Could you check a few things on this model? Use its own coordinates, in mm. Face numbers are marked on the shaded views. A direction names the side the tool comes from. Give positions to 0.01 mm unless a question says otherwise; leave off trailing zeros. Write each loop counter-clockwise with the first axis right and the second up, starting at its lowest first coordinate (ties: lowest second). Pieces come first, ordered by that corner, then holes. Notation, with made-up numbers: (33.5, 25) - (77.5, 25) arc R27 cw to (77.5, 42) - close; hole circle Ø7 at (29.25, 32.5). An arc over 180 degrees is marked (long way). Use one line per item in the form item = value.
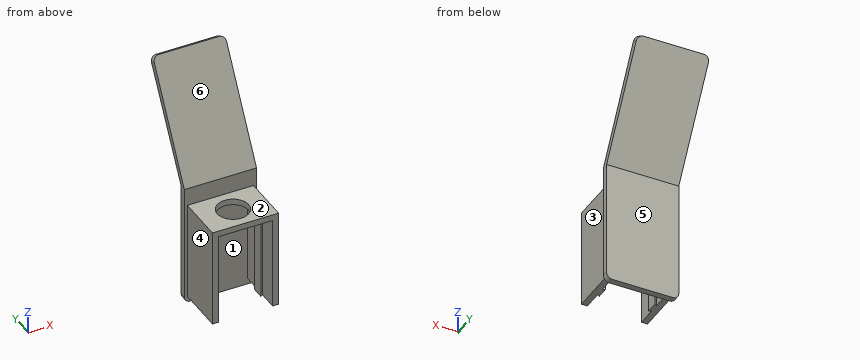
```python
from build123d import *

# Parameters (mm, degrees)
F0_W      = 5
F0_H      = 102
F1_DEPTH  = 60
F2_W      = 5
F2_H      = 82
F3_DEPTH  = 40
F4_R      = 5
F5_W      = 45
F5_H      = 5
F6_DEPTH  = 40
F7_R      = 13
F8_DEPTH  = 25
F10_DEPTH = 77
F12_DEPTH = 77


with BuildPart() as f1:
    # F0 (on Right) → F1 (new body)
    with BuildSketch(Plane.YZ):
        Polygon((47.787035, 88.742403), (-2.5, 0), (2.5, 0), (52.248346, 86.166664), align=None)
        with Locations((0, -51)):
            Rectangle(F0_W, F0_H)
    extrude(amount=F1_DEPTH)

    # F2 (on face) → F3 (join)
    with BuildSketch(Plane.XZ.offset(2.5)):
        with Locations((5, -56)):
            Rectangle(F2_W, F2_H)
        with Locations((55, -56)):
            Rectangle(F2_W, F2_H)
    extrude(amount=F3_DEPTH)

    # F4
    f4_edges = [f1.edges().sort_by_distance(p)[0] for p in [
        (0, 50.017691, 87.454534),
        (60, 50.017691, 87.454534),
        (60, 0, -102),
        (0, 0, -102),
    ]]
    fillet(f4_edges, radius=F4_R)

    # F5 (on face) → F6 (join)
    with BuildSketch(Plane.XZ.offset(2.5)):
        with Locations((30, -17.5)):
            Rectangle(F5_W, F5_H)
    extrude(amount=F6_DEPTH)

    # F7 (on face) → F8 (cut)
    with BuildSketch(Plane.XY.offset(-15)):
        with Locations((30, -22.5)):
            Circle(F7_R)
    extrude(amount=-F8_DEPTH, mode=Mode.SUBTRACT)

    # F9 (on face) → F10 (join, through all)
    with BuildSketch(Plane(origin=(0, 0, -97), x_dir=(1, 0, 0), z_dir=(0, 0, -1))):
        Polygon((9.5, 27.5), (7.5, 26.5), (7.5, 18.5), (9.5, 17.5), (9.5, 18.5), (9.5, 26.5), align=None)
    extrude(amount=-F10_DEPTH)

    # F11 (on face) → F12 (join, through all)
    with BuildSketch(Plane(origin=(0, 0, -97), x_dir=(1, 0, 0), z_dir=(0, 0, -1))):
        Polygon((52.5, 18.5), (52.5, 26.5), (50.5, 27.5), (50.5, 26.5), (50.5, 18.5), (50.5, 17.5), align=None)
    extrude(amount=-F12_DEPTH)


solid = f1.part
```
1. Imagine slicing it at C-C, the plane z = -87. List the corners of the cut face in (x, y) for me, and give its area (3 significant figures).
Response values:
outline = (0, -2.5) - (2.5, -2.5) - (2.5, -42.5) - (7.5, -42.5) - (7.5, -26.5) - (9.5, -27.5) - (9.5, -17.5) - (7.5, -18.5) - (7.5, -2.5) - (52.5, -2.5) - (52.5, -18.5) - (50.5, -17.5) - (50.5, -27.5) - (52.5, -26.5) - (52.5, -42.5) - (57.5, -42.5) - (57.5, -2.5) - (60, -2.5) - (60, 2.5) - (0, 2.5) - close
area = 736 mm²
2. If we mould it in two halves opening along X, with no side actions, what happens to the marked faces 1, 2 and 3? For each: pulls with the +X half, pulls with the -X half, needs draft (parallel to the pull), parting line crosses it, or undercut.
Response values:
face_1 = undercut
face_2 = needs draft
face_3 = pulls with the +X half
3. For pin 1 (12 mm diameter, centred on y = -17, z = -58.5, fed in from -X); pin 2 (2 mm diameter, centred on x = 6, y = -19.5, fed in from -Z); pin 3 (8 mm diameter, centred on y = -22.5, z = -47, fed in from +X), each with a flat end and sliding along its axis, tell me the tip position at first contact or that it passes through.
Response values:
pin_1 = 2.5
pin_2 = -97
pin_3 = 57.5
4. Imagine slicing it at A-A, the plane y = -22.5. List the corners of the cut face in (x, z) for me, and give its area (3 significant figures).
Response values:
outline = (2.5, -97) - (9.5, -97) - (9.5, -20) - (17, -20) - (17, -15) - (2.5, -15) - close; (43, -20) - (50.5, -20) - (50.5, -97) - (57.5, -97) - (57.5, -15) - (43, -15) - close
area = 1,220 mm²
5. Imagine slicing it at B-B, the plane x = 31.5. List the corners of the cut face in (y, z) for me.
Response values:
outline = (-42.5, -20) - (-35.41, -20) - (-35.41, -15) - (-42.5, -15) - close; (-9.59, -20) - (-2.5, -20) - (-2.5, -102) - (2.5, -102) - (2.5, 0) - (52.25, 86.17) - (47.79, 88.74) - (-2.5, 0) - (-2.5, -15) - (-9.59, -15) - close
6. If I drill on line 1 (Y direction, x = 30, z = -16.05); line 2 (X direction, y = -22, z = -17); line 3 (Y direction, x = 47.5, z = -3), over which ranges is the centre line in solid material (lowest first)? Write a range as from..to.
Response values:
line_1 = -42.5..-35.5, -9.5..2.5
line_2 = 2.5..17.01, 42.99..57.5
line_3 = -2.5..2.5
7. Imagine slicing it at D-D, the plane x = 20. List the corners of the cut face in (y, z) for me, and give its area (3 significant figures).
Response values:
outline = (-42.5, -20) - (-30.81, -20) - (-30.81, -15) - (-42.5, -15) - close; (-14.19, -20) - (-2.5, -20) - (-2.5, -102) - (2.5, -102) - (2.5, 0) - (52.25, 86.17) - (47.79, 88.74) - (-2.5, 0) - (-2.5, -15) - (-14.19, -15) - close
area = 1,110 mm²
8. Which directions (+Z, -Z, +X, -X, +Y, -Y) give clear straight access to the entire face, cutting with the end or side of a thin tool? Please do the marked faces 4, 5 and 6.
Response values:
face_4 = +Z, -Z, -X, -Y
face_5 = -Z, +X, -X, +Y
face_6 = +Z, +X, -X, -Y
